from build123d import *

# Parameters (mm, degrees)
SKETCH_1_W           = 42.3
SKETCH_1_H           = 10
EXTRUDE_3_DEPTH      = 240
SKETCH_2_W           = 42.3
SKETCH_2_H           = 140
CUT_EXTRUDE_1_DEPTH  = 100
SKETCH_3_W           = 42.7
SKETCH_3_H           = 240
EXTRUDE_4_DEPTH      = 140
CUT_EXTRUDE_2_REACH  = 287.139
SKETCH_4_W           = 32.7
SKETCH_4_H           = 120
SKETCH_7_W           = 32.7
SKETCH_7_H           = 140
CUT_EXTRUDE_6_DEPTH  = 100
FILLET_2_R           = 70
SKETCH_6_R           = 35
SKETCH_6_R_2         = 1.75
CUT_EXTRUDE_7_DEPTH  = 10
SKETCH_5_R           = 30
SKETCH_5_R_2         = 1.75
CUT_EXTRUDE_8_DEPTH  = 10
SKETCH_8_W           = 10
SKETCH_8_H           = 140
EXTRUDE_5_DEPTH      = 110
FILLET_4_R           = 60
SKETCH_17_R          = 25
CUT_EXTRUDE_13_DEPTH = 139
CUT_EXTRUDE_14_DEPTH = 110
SKETCH_19_R          = 37.5
CUT_EXTRUDE_15_DEPTH = 14


with BuildPart() as part:
    # 草图1 → 凸台-拉伸3 (new body)
    with BuildSketch(Plane.XY):
        with Locations((-15.094230769, 5.936538462)):
            Rectangle(SKETCH_1_W, SKETCH_1_H)
        Polygon((-36.244230769, 0.936538462), (-36.244230769, 10.936538462), (-41.244230769, 10.936538462), (-41.244230769, -129.063461538), (-36.244230769, -129.063461538), (-36.244230769, -119.063461538), align=None)
        Polygon((16.055769231, 10.936538462), (6.055769231, 10.936538462), (6.055769231, 0.936538462), (6.055769231, -119.063461538), (6.055769231, -129.063461538), (16.055769231, -129.063461538), align=None)
        with Locations((-15.094230769, -124.063461538)):
            Rectangle(SKETCH_1_W, SKETCH_1_H)
    extrude(amount=EXTRUDE_3_DEPTH)

    # 草图2 → 切除-拉伸1 (cut)
    with BuildSketch(Plane.XY.offset(240)):
        with Locations((-15.094230769, -59.063461538)):
            Rectangle(SKETCH_2_W, SKETCH_2_H)
    extrude(amount=-CUT_EXTRUDE_1_DEPTH, mode=Mode.SUBTRACT)

    # 草图3 → 凸台-拉伸4 (add)
    with BuildSketch(Plane.XZ.offset(129.063461538)):
        with Locations((-62.594230769, 120)):
            Rectangle(SKETCH_3_W, SKETCH_3_H)
    extrude(amount=-EXTRUDE_4_DEPTH)

    # 草图4 → 切除-拉伸2 (cut, up to next)
    with BuildSketch(Plane.XY.offset(240), mode=Mode.PRIVATE) as cut_extrude_2_sk1:
        with Locations((-57.594230769, -59.063461538)):
            Rectangle(SKETCH_4_W, SKETCH_4_H)
    cut_extrude_2_tool1 = extrude(cut_extrude_2_sk1.sketch, amount=-CUT_EXTRUDE_2_REACH, mode=Mode.PRIVATE) & part.part
    add(cut_extrude_2_tool1.solids().sort_by_distance((-57.594231, -59.063462, 240))[0], mode=Mode.SUBTRACT)

    # 草图7 → 切除-拉伸6 (cut)
    with BuildSketch(Plane.XY.offset(240)):
        with Locations((-57.594230769, -59.063461538)):
            Rectangle(SKETCH_7_W, SKETCH_7_H)
    extrude(amount=-CUT_EXTRUDE_6_DEPTH, mode=Mode.SUBTRACT)

    # 圆角2
    fillet_2_edges = [part.edges().sort_by_distance(p)[0] for p in [
        (11.055769231, 10.936538462, 240),
        (-38.744230769, 10.936538462, 240),
        (-78.944230769, 10.936538462, 240),
        (11.055769231, -129.063461538, 240),
        (-38.744230769, -129.063461538, 240),
        (-78.944230769, -129.063461538, 240),
    ]]
    fillet(fillet_2_edges, radius=FILLET_2_R - 0.0001)  # a hair under: the kernel refuses the full size

    # 草图6 → 切除-拉伸7 (cut)
    with BuildSketch(Plane.ZY.offset(41.244230769)):
        with Locations((192, -59.063461538)):
            Circle(SKETCH_6_R)
        with Locations((149.5, -59.063461538)):
            Circle(SKETCH_6_R_2)
        with Locations((161.9479618, -29.011423338)):
            Circle(SKETCH_6_R_2)
        with Locations((192, -16.563461538)):
            Circle(SKETCH_6_R_2)
        with Locations((222.0520382, -29.011423338)):
            Circle(SKETCH_6_R_2)
        with Locations((234.5, -59.063461538)):
            Circle(SKETCH_6_R_2)
        with Locations((222.0520382, -89.115499739)):
            Circle(SKETCH_6_R_2)
        with Locations((192, -101.563461538)):
            Circle(SKETCH_6_R_2)
        with Locations((161.9479618, -89.115499739)):
            Circle(SKETCH_6_R_2)
    extrude(amount=-CUT_EXTRUDE_7_DEPTH, mode=Mode.SUBTRACT)

    # 草图5 → 切除-拉伸8 (cut)
    with BuildSketch(Plane.ZY.offset(83.944230769)):
        with Locations((192, -59.063461538)):
            Circle(SKETCH_5_R)
        with Locations((161.9479618, -29.011423338)):
            Circle(SKETCH_5_R_2)
        with Locations((149.5, -59.063461538)):
            Circle(SKETCH_5_R_2)
        with Locations((161.9479618, -89.115499739)):
            Circle(SKETCH_5_R_2)
        with Locations((192, -101.563461538)):
            Circle(SKETCH_5_R_2)
        with Locations((222.0520382, -89.115499739)):
            Circle(SKETCH_5_R_2)
        with Locations((234.5, -59.063461538)):
            Circle(SKETCH_5_R_2)
        with Locations((222.0520382, -29.011423338)):
            Circle(SKETCH_5_R_2)
        with Locations((192, -16.563461538)):
            Circle(SKETCH_5_R_2)
    extrude(amount=-CUT_EXTRUDE_8_DEPTH, mode=Mode.SUBTRACT)

    # 草图8 → 凸台-拉伸5 (add)
    with BuildSketch(Plane(origin=(0, 0, 0), x_dir=(-1, 0, 0), z_dir=(0, 0, -1))):
        with Locations((-11.055769231, -59.063461538)):
            Rectangle(SKETCH_8_W, SKETCH_8_H)
        with Locations((78.944230769, -59.063461538)):
            Rectangle(SKETCH_8_W, SKETCH_8_H)
    extrude(amount=EXTRUDE_5_DEPTH)

    # 圆角4
    fillet_4_edges = [part.edges().sort_by_distance(p)[0] for p in [
        (11.055769231, 10.936538462, -110),
        (11.055769231, -129.063461538, -110),
        (-78.944230769, -129.063461538, -110),
        (-78.944230769, 10.936538462, -110),
    ]]
    fillet(fillet_4_edges, radius=FILLET_4_R)

    # 草图17 → 切除-拉伸13 (cut)
    with BuildSketch(Plane.ZY.offset(83.944230769)):
        with Locations(Location((192, -59.063461538, 0), (0, 0, 180))):
            Circle(SKETCH_17_R)
    extrude(amount=-CUT_EXTRUDE_13_DEPTH, mode=Mode.SUBTRACT)

    # 草图18 → 切除-拉伸14 (cut)
    with BuildSketch(Plane(origin=(16.055769231, 0, 0), x_dir=(0, 0, -1), z_dir=(1, 0, 0))):
        with BuildLine():
            Line((-60, 86.355512133), (-60, 10.936538462))
            Line((-60, 10.936538462), (50, 10.936538462))
            ThreePointArc((50, 10.936538462), (92.426406871, -6.637054667), (110, -49.063461538))
            Line((110, -49.063461538), (110, -69.063461538))
            ThreePointArc((110, -69.063461538), (92.426406871, -111.48986841), (50, -129.063461538))
            Line((50, -129.063461538), (-60, -129.063461538))
            Line((-60, -129.063461538), (-60, -152.364477091))
            Line((-60, -152.364477091), (264.503295558, -152.364477091))
            Line((264.503295558, -152.364477091), (264.503295558, 86.355512133))
            Line((264.503295558, 86.355512133), (-60, 86.355512133))
        make_face()
        with BuildLine():
            Line((50, 10.936538462), (-60, 10.936538462))
            Line((-60, 10.936538462), (-60, -129.063461538))
            Line((-60, -129.063461538), (50, -129.063461538))
            ThreePointArc((50, -129.063461538), (92.426406871, -111.48986841), (110, -69.063461538))
            Line((110, -69.063461538), (110, -49.063461538))
            ThreePointArc((110, -49.063461538), (92.426406871, -6.637054667), (50, 10.936538462))
        make_face()
    extrude(amount=-CUT_EXTRUDE_14_DEPTH, mode=Mode.SUBTRACT)

    # 镜向2: part across plane


with BuildPart() as part_1:
    add(part.part)
    add(part.part.mirror(Plane(origin=(-93.944230769, 0, 60), x_dir=(1, 0, 0), z_dir=(0, 0, 1))))

    # 草图19 → 切除-拉伸15 (cut)
    with BuildSketch(Plane(origin=(16.055769231, 0, 0), x_dir=(0, 0, -1), z_dir=(1, 0, 0))):
        with Locations((72, -59.063461538)):
            Circle(SKETCH_19_R)
    extrude(amount=-CUT_EXTRUDE_15_DEPTH, mode=Mode.SUBTRACT)


solid = part_1.part
Design review of the part built by this model. Coordinates are the model's own, in mm. A direction names the side the tool comes from. Round coordinates to 2 decimals unless told otherwise and drop trailing zeros. Write each loop counter-clockwise with the first axis right and the second up, starting at its lowest first coordinate (ties: lowest second). Pieces come first, ordered by that corner, then holes. Notation, with made-up numbers: M 13.5,65 L 18.5,65 A25 cw 18.5,87 Z; hole C -15.5,77.25 d5. An arc over 180 degrees is marked long. One line per item, written item: value. Start each with the question number.
1. For faces 1 (the face through (-58, 0.937, 59)), 2 (the face through (-33, -129.063, 58)), list the 3-axis set-ups (+Z, -Z, +X, -X, +Y, -Y) from which the entire face can be reached by the end or side of a thin tool; tool diameter is ignored.
2. To check wall thickness, follow probe 1 along X at (y, z) = (-6, 148); probe 2 along Y at (x, z) = (-30.5, 35); probe 3 along X at (y, z) = (-25, -61.5). State the ranges of each line that lie inside material, in increasing order. Write a range as from..to.
3. Take a section at C-C on y = -114.5. State the section outline as (x, z) points.
4. Take a section at A-A on x = -52.5. State the section outline as (y, z) points.
5. Clearance check with flat-ended pins moving along their axes: P1, Ø3, axis at y = -101.56, z = -72, coming from the -X side; P2, Ø11, axis at x = -17, y = -121.5, coming from the +Z side; P3, Ø11, axis at x = -55.5, y = 8, coming from the -Z side. State where each tip first meets the part, or that it passes through.
6. Draft analysis for pull direction Z (two halves, no side actions). For faces 3 (the face through (-78.87, -109.1, 218.95)), 4 (the face through (-15, -124, -20)), 5 (the face through (-15, -119.063, 61)), 6 (the face through (10.986, -66.573, 168.154)), state which applies: pulls with the +Z half, pulls with the -Z half, needs draft (parallel to the pull), parting line crosses it, or undercut.
7. Take a section at D-D on z = 209.5. State the section outline as (x, y) points, then the cut area to 3 significant figures.
8. Take a section at B-B on z = 123. State the section outline as (x, y) points.
Computed:
1. face 1: +Z, -Z
1. face 2: +Z, -Z, +X, -X, -Y
2. probe 1: x = -83.94..-73.94, -41.24..-36.24, 6.06..16.06
2. probe 2: y = -129.06..-119.06, 0.94..10.94
2. probe 3: x = -83.94..-73.94, -41.24..-36.24
3. outline: M -83.94,-92.74 L -73.94,-92.74 L -73.94,212.74 L -83.94,212.74 Z; M -41.24,-92.74 L -36.24,-92.74 L -36.24,212.74 L -41.24,212.74 Z; M 6.06,-92.74 L 16.06,-92.74 L 16.06,212.74 L 6.06,212.74 Z
4. outline: M -129.06,-20 L -119.06,-20 L -119.06,140 L -129.06,140 Z; M 0.94,-20 L 10.94,-20 L 10.94,140 L 0.94,140 Z
5. P1: stops at x = 6.06
5. P2: stops at z = 140
5. P3: stops at z = -20
6. face 3: pulls with the +Z half
6. face 4: pulls with the -Z half
6. face 5: needs draft
6. face 6: undercut
7. outline: M -83.94,-116.85 L -73.94,-116.85 L -73.94,-83.43 L -83.94,-83.43 Z; M -83.94,-34.7 L -73.94,-34.7 L -73.94,-1.27 L -83.94,-1.27 Z; M -41.24,-116.85 L -36.24,-116.85 L -36.24,-89.37 L -41.24,-89.37 Z; M -41.24,-28.75 L -36.24,-28.75 L -36.24,-1.27 L -41.24,-1.27 Z; M 6.06,-116.85 L 16.06,-116.85 L 16.06,-76.92 L 6.06,-76.92 Z; M 6.06,-41.21 L 16.06,-41.21 L 16.06,-1.27 L 6.06,-1.27 Z
7. area: 1,740 mm²
8. outline: M -83.94,-129.06 L 16.06,-129.06 L 16.06,10.94 L -83.94,10.94 Z; hole M -73.94,-119.06 L -41.24,-119.06 L -41.24,0.94 L -73.94,0.94 Z; hole M -36.24,-119.06 L 6.06,-119.06 L 6.06,0.94 L -36.24,0.94 Z
